The listing builds one solid part. Answer for the finished solid, in the listing's coordinates (mm). A direction names the side the tool comes from. Coordinates: 2 decimals unless noted, no trailing zeros. Order: outer loops, then holes, each group sorted by start corner. A loop starts at its lowest first (then second) coordinate and runs counter-clockwise, first axis right, second up. Notation, with made-up numbers: (-29, 71) -> (-3, 71) arc R19 cw to (-3, 86) -> close; hole circle Ø5 at (-38, 21). An arc over 180 degrees is marked (long way). Answer in a Markdown table with one row per item.
Autodesk Inventor part; units mm, degrees
ref_plane "YZ Plane" through (0, 0, 0) normal (1, 0, 0) x (0, 1, 0)
ref_plane "XZ Plane" through (0, 0, 0) normal (0, 1, 0) x (-1, 0, 0)
ref_plane "XY Plane" through (0, 0, 0) normal (0, 0, 1) x (1, 0, 0)
sketch "Sketch1" plane through (0, 0, 0) normal (0, 1, 0) x (-1, 0, 0)
  line L0 (-1.7898, -3.1) -> (-3.5796, 0)
  line L1 (-3.5796, 0) -> (-1.7898, 3.1)
  line L2 (-1.7898, 3.1) -> (1.7898, 3.1)
  line L3 (1.7898, 3.1) -> (3.5796, 0)
  line L4 (3.5796, 0) -> (1.7898, -3.1)
  line L5 (1.7898, -3.1) -> (-1.7898, -3.1)
  circle A0 centre (0, 0) radius 5
  spline S0 degree 2 poles (1.7898, 3.1) (0, 2.8) (-1.7898, 3.1) knots 0 0 0 1 1 1
  spline S1 degree 2 poles (-1.7898, 3.1) (-2.4249, 1.4) (-3.5796, 0) knots 0 0 0 1 1 1
  spline S2 degree 2 poles (-3.5796, 0) (-2.4249, -1.4) (-1.7898, -3.1) knots 0 0 0 1 1 1
  spline S3 degree 2 poles (-1.7898, -3.1) (0, -2.8) (1.7898, -3.1) knots 0 0 0 1 1 1
  spline S4 degree 2 poles (1.7898, -3.1) (2.4249, -1.4) (3.5796, 0) knots 0 0 0 1 1 1
  spline S5 degree 2 poles (3.5796, 0) (2.4249, 1.4) (1.7898, 3.1) knots 0 0 0 1 1 1
  point P0 (0, 0)
  point P1 (0, 0)
  point P2 (0, -3.1)
  point P3 (0, 2.95)
  point P4 (0, 3.1)
  point P5 (-2.5548, 1.475)
  point P6 (-2.5548, -1.475)
  point P7 (0, -2.95)
  point P8 (2.5548, -1.475)
  point P9 (2.5548, 1.475)
  point P10 (1.7898, 3.1)
  point P11 (1.7898, 3.1)
  point P12 (1.7898, 3.1)
  dimension "d0" = 3.1
  dimension "d1" = 10
  dimension "d27" = 0.15
  dimension "d30" = 360
extrude "Extrusion1" add sketch "Sketch1" along normal blind 8 contours S3 L5 | L0 S2 | L1 S1 | S4 L4 | L2 S0 | S5 L3 | A0
sketch "Sketch2" plane through (0, 8, 0) normal (0, 1, 0) x (1, 0, 0)
  circle A0 centre (0, 0) radius 0.5
  circle A1 centre (0, 0) radius 5
  circle A2 centre (0, 0) radius 5
  dimension "d4" = 1
sketch "Sketch5" plane through (0, 0, 0) normal (0, 0, 1) x (1, 0, 0)
  line L0 (5, 8) -> (-5, 8)
  line L1 (5, 8) -> (5, 11.5)
  line L2 (5, 11.5) -> (3.5, 11.5)
  line L3 (5, 8) -> (0.5, 8)
  line L4 (0.5, 8) -> (3.5, 11.5)
  line L5 (0, 8) -> (0, 11)
  point P0 (0, 0)
  dimension "d20" = 3.5
  dimension "d21" = 1.5
  dimension "d22" = 4.5
  dimension "d23" = 3
revolve "Revolution1" add sketch "Sketch5" angle 360 about axis through (0, 8, 0) along (0, 1, 0)
sketch "Sketch7" plane through (0, 11.5, 0) normal (0, 1, 0) x (1, 0, 0)
  circle A0 centre (0, 0) radius 0.5
  circle A1 centre (0, 0) radius 3.5
  circle A2 centre (0, 0) radius 5
extrude "Extrusion2" add sketch "Sketch7" along normal blind 8 contours A2
properties part number "seegoals_adapter_puller_tool_v1"
(1) A cutting plane is placed at A-A, the plane z = -4. Determine the outline of the cut face in (x, y), then the cut area to 3 significant figures.
Check values:
| item | result |
|---|---|
| outline | (-3, 0) -> (3, 0) -> (3, 19.5) -> (-3, 19.5) -> close |
| area | 117 mm² |
(2) Find the intervals of material crossed by line 1 along X through (y, z) = (13.5, 0); line 2 along X through (y, z) = (14, 1.75), in increasing order. Write a range as from..to.
Check values:
| item | result |
|---|---|
| line 1 | -5..-3.5, 3.5..5 |
| line 2 | -4.68..-3.03, 3.03..4.68 |
(3) For a pull along X with two mould halves and no side action, classify faces 3 (the flat face through (2.2, 19.5, 3.3)), 4 (the cylindrical face through (3.233, 15.444, -1.341)), 5 (the cylindrical face through (0, 7, -5)) as released by +X, released by -X, zero draft, split by the parting line, or undercut.
Check values:
| item | result |
|---|---|
| face 3 | zero draft |
| face 4 | undercut |
| face 5 | split by the parting line |
(4) Flat-ended cylindrical pins translate along their axes: pin 1 (3 mm diameter, centred on y = 5.5, z = -3.5, fed in from +X); pin 2 (3 mm diameter, centred on x = 1, z = -1.5, fed in from +Y); pin 3 (1.5 mm diameter, centred on x = 0.5, z = -1.5, fed in from -Y). Find the tip coordinate at first contact, or state that the pin passes through.
Check values:
| item | result |
|---|---|
| pin 1 | x = 4.58 |
| pin 2 | y = 11.27 |
| pin 3 | y = 8 |
(5) Which of the six approach directions +Z, -Z, +X, -X, +Y, -Y give full straight-line access (tool end or side, diameter ignored) to faces 1 (the flat face through (0, 8, 1)), 2 (the conical face through (-0.22, 8.61, 1))?
Check values:
| item | result |
|---|---|
| face 1 | -Y |
| face 2 | +Y |
(6) A cutting plane is placed at B-B, the plane y = 14.75. Determine the outline of the cut face in (x, z), then the cut area to 3 significant figures.
Check values:
| item | result |
|---|---|
| outline | circle Ø10 at (0, 0); hole circle Ø7 at (0, 0) |
| area | 40.1 mm² |
